The model under review builds one solid part; all positions refer to its coordinate system, in mm. A direction names the side the tool comes from. Give positions to 0.01 mm unless a question says otherwise; leave off trailing zeros. Write each question's results on one line, items separated by ' | '. Start each with the question number.
Q1. We need section A-A (z = -7). Give the number of separate pieces and of enclosed holes in the cut face, plus the area to 3 significant figures.
Q2. Machinability: for faces 1 (the face through (12, -11, -8)), 2 (the face through (43, 0, -4)), which of the approach directions +Z, -Z, +X, -X, +Y, -Y give a long, thin tool a straight path to every point of the face, cutting with its end or side? Answer none if there is none.
Q3. Wall thickness on L1, parallel to X at y = -13, z = -5.25; L2, parallel to X at y = -24, z = -2.75; L3, parallel to Y at x = 17, z = -2.75: over which ranges is each line inside the solid? List them lowest first. Write a range as [from, to].
Q4. Insertion check: pin 1 Ø0.6 at (x, z) = (42.5, -3) entering from -Y; pin 2 Ø1.5 at (y, z) = (-10, -3.5) entering from +X; pin 3 Ø4 at (x, z) = (32, -3) entering from -Y; pin 4 Ø1.4 at (x, y) = (3, -12.5) entering from -Z. Each pin has a flat end and moves straight along its axis. Give the tip position at first contact, or say it passes through.
Q5. Mouldability with a two-part tool opening along X and no side actions: class faces 3 (the face through (0.86, -39.1, -4.06)), 4 (the face through (8, 0, -4)), 5 (the face through (13.13, -3.49, -4.06)) as released by +X, released by -X, zero draft, split by the parting line, or undercut.
from build123d import *

# Parameters (mm, degrees)
EXTRUDE_641_DEPTH = 8
FILLET_2_R        = 3
FILLET_3_RADIUS   = 0.75
FILLET_3_LENGTH   = 8
HOLE_WIZARD_M2_D  = 1.6
FILLET_4_R        = 3


with BuildPart() as part:
    # Model → Extrude 641 (new body)
    with BuildSketch(Plane.XY):
        with BuildLine():
            Line((0, 0), (13, 0))
            Line((13, 0), (14.5, 1.5))
            Line((14.5, 1.5), (44, 1.5))
            Line((44, 1.5), (44, 0))
            Line((44, 0), (42, 0))
            add(Edge.make_bspline(
                [(3, -40), (3, -11.686704979), (28.988478702, 0), (42, 0)],
                knots=[0, 0, 0, 0, 0.938491694, 0.938491694, 0.938491694, 0.938491694], degree=3))
            Line((3, -40), (0, -40))
            Line((0, -40), (0, 0))
        make_face()
    extrude(amount=-EXTRUDE_641_DEPTH)

    # Скругление2
    fillet_2_edges = [part.edges().sort_by_distance(p)[0] for p in [
        (0, 0, -4),
    ]]
    fillet(fillet_2_edges, radius=FILLET_2_R)

    # Скругление3: full round fillet: the end face becomes a half cylinder, R = half its width
    fillet_3_face = Plane((44, 0.75, -4), x_dir=(0, 0, 1), z_dir=(1, 0, 0))  # on the end face: x along it, z out of the body
    fillet_3_slab = fillet_3_face.offset(-FILLET_3_RADIUS / 2) * Box(FILLET_3_LENGTH, 2 * FILLET_3_RADIUS, FILLET_3_RADIUS, mode=Mode.PRIVATE)  # the body's end, R deep
    fillet_3_round = Plane((43.25, 0.75, -4), x_dir=(1, 0, 0), z_dir=(0, 0, 1)) * Cylinder(FILLET_3_RADIUS, FILLET_3_LENGTH, mode=Mode.PRIVATE)  # its axis R under the face
    add(fillet_3_slab - fillet_3_round, mode=Mode.SUBTRACT)

    # Крепление M2 (through all)
    with Locations(Plane.XY):
        with Locations((3, -12.5), (12.5, -3)):
            Hole(HOLE_WIZARD_M2_D / 2)

    # Скругление4
    fillet_4_edges = [part.edges().sort_by_distance(p)[0] for p in [
        (0, -40, -4),
    ]]
    fillet(fillet_4_edges, radius=FILLET_4_R - 0.0001)  # a hair under: the kernel refuses the full size


solid = part.part
Output:
1) separate pieces: 1 | enclosed holes: 2 | area: 505 mm2
2) face 1: -Z, +X, -X, +Y, -Y | face 2: +Z, -Z, +X, -Y
3) L1: [0, 2.38], [3.62, 13.63] | L2: [0, 6.21] | L3: [-9.89, 1.5]
4) pin 1: y = 0 | pin 2: x = 17.79 | pin 3: y = -2.42 | pin 4: through
5) face 3: released by -X | face 4: zero draft | face 5: undercut
